from build123d import *

# Parameters (mm, degrees)
F0_W     = 5.7972974144
F0_H     = 5.9
F0_H_2   = 19.1
F1_DEPTH = 12.5
F3_D     = 4.4
F3_DEPTH = 14.1
F3_TIP   = 1.3218933619
F4_DEPTH = 3.625


with BuildPart() as f1:
    # F0 (on Front) → F1 (new body, symmetric)
    with BuildSketch(Plane.XZ):
        with Locations((-4.0329019539, -17.188550967)):
            Rectangle(F0_W, F0_H)
        with BuildLine():
            ThreePointArc((29.8217841377, -15.618166969), (29.3859073845, -15.4145662467), (28.9485841576, -15.214091327))
            ThreePointArc((28.9485841576, -15.214091327), (29.3823237659, -15.4223103801), (29.8217841377, -15.618166969))
        make_face()
        with Locations((-4.0329019539, 25.311449033)):
            Rectangle(F0_W, F0_H_2)
        with BuildLine():
            Line((19.5255004201, 0), (-1.1342532467, 0))
            Line((-1.1342532467, 0), (-1.1342532467, -9.2409374192))
            ThreePointArc((-1.1342532467, -9.2409374192), (14.2525091884, -10.4882457176), (28.9485841576, -15.214091327))
            ThreePointArc((28.9485841576, -15.214091327), (22.072081358, -8.9479478378), (19.5255004201, 0))
        make_face()
        with BuildLine():
            Line((23.5255004201, 0), (19.5255004201, 0))
            ThreePointArc((19.5255004201, 0), (22.072081358, -8.9479478378), (28.9485841576, -15.214091327))
            ThreePointArc((28.9485841576, -15.214091327), (29.3859073845, -15.4145662467), (29.8217841377, -15.618166969))
            ThreePointArc((29.8217841377, -15.618166969), (45.8723890611, -14.1878546071), (53.5125784245, 0))
            Line((53.5125784245, 0), (49.5125784245, 0))
            ThreePointArc((49.5125784245, 0), (36.5190394223, -12.9935390022), (23.5255004201, 0))
        make_face()
        Polygon((-1.1342532467, 15.761449033), (-6.9315506611, 15.761449033), (-6.9315506611, -14.238550967), (-1.1342532467, -14.238550967), (-1.1342532467, -9.2409374192), (-1.1342532467, 0), align=None)
    extrude(amount=F1_DEPTH, both=True)

    # F3
    with Locations(Plane(origin=(-6.9315506611, 0, 0), x_dir=(0, -1, 0), z_dir=(-1, 0, 0))):
        with Locations((0, 15.79714939), (0, -14.253873378)):
            Hole(F3_D / 2, depth=F3_DEPTH)
            with Locations((0, 0, -(F3_DEPTH + F3_TIP / 2))):  # 118° drill point
                Cone(0, F3_D / 2, F3_TIP, mode=Mode.SUBTRACT)

    # F0 (on Front) → F4 (join, symmetric)
    with BuildSketch(Plane.XZ):
        Polygon((-10.9315506611, 34.861449033), (-6.9315506611, 34.861449033), (-1.1342532467, 34.861449033), (-6.9315506611, 60.7583903916), (-14.991494827, 60.7583903916), (-14.991494827, 56.861449033), (-10.9315506611, 56.861449033), align=None)
    extrude(amount=F4_DEPTH, both=True)


solid = f1.part
Here's how the part is built. I have some questions about the finished solid (model axes, mm). A direction names the side the tool comes from. Coordinates: 2 decimals unless noted, no trailing zeros. Loops run counter-clockwise (first coordinate to the right, second up) from the corner with the lowest first, then second, coordinate; pieces in that order, holes last.
1. Imagine slicing it at C-C, the plane x = -3. Please give me the cut outline in (y, z) (3 decimals), and give its area (3 significant figures).
2. For faces 4 (the flat face through (-1.134, -3, 17)), 5 (the flat face through (-6.932, 0, 8)), 6 (the flat face through (-8, -3.625, 48)), which set-ups out of +Z, -Z, +X, -X, +Y, -Y let a thin tool reach every point of the face, with its end or its side?
3. If we mould it in two halves opening along Z, with no side actions, what happens to faces 1 (the flat face through (-4, 0, -20.139)), 2 (the flat face through (-1.134, 0, -17)), 3 (the cylindrical face through (-3.992, -0.286, 17.978))? For each: pulls with the +Z half, pulls with the -Z half, needs draft (parallel to the pull), parting line crosses it, or undercut.
4. Imagine slicing it at A-A, the plane y = 0. Please give me the cut outline in (x, z).
5. For P1, Ø1, axis at x = 42.5, y = 3.5, coming from the -Z side; P2, Ø1.7, axis at x = -4.5, y = 6, coming from the +Z side; P3, Ø3, axis at x = 51, y = 3, coming from the +Z side, each with a flat end and sliding along its axis, tell me the tip position at first contact or that it passes through.
6. I need wall thicknesses on L1, parallel to X at y = 5, z = 12; L2, parallel to Y at x = -4.5, z = 49.5 (3 decimals); L3, parallel to X at y = -5.75, z = -7. Which ranges of each line are inside material? Lowest first, please.
7. Imagine slicing it at D-D, the plane z = 36. Please give me the cut outline in (x, y) (3 decimals), and give its area (3 significant figures).
8. Imagine slicing it at B-B, the plane y = 7.5. Please give me the cut outline in (x, z), and give its area (3 significant figures).
Taken from the geometry:
1. outline: (-12.5, -20.139) - (12.5, -20.139) - (12.5, 34.861) - (3.625, 34.861) - (3.625, 43.196) - (-3.625, 43.196) - (-3.625, 34.861) - (-12.5, 34.861) - close; hole circle Ø4.4 at (0, -14.254); hole circle Ø4.4 at (0, 15.797)
1. area: 1,410 mm2
2. face 4: +Z, +X, +Y, -Y
2. face 5: -Z, -X, +Y, -Y
2. face 6: +Z, +X, -X, -Y
3. face 1: pulls with the -Z half
3. face 2: needs draft
3. face 3: undercut
4. outline: (-14.99, 56.86) - (-10.93, 56.86) - (-10.93, 34.86) - (-6.93, 34.86) - (-6.93, 18) - (-1.13, 18) - (-1.13, 34.86) - (-6.93, 60.76) - (-14.99, 60.76) - close; (-6.93, -20.14) - (-1.13, -20.14) - (-1.13, -16.45) - (-6.93, -16.45) - close; (-6.93, -12.05) - (-1.13, -12.05) - (-1.13, -9.24) arc R67.2 cw to (28.95, -15.21) arc R16.99 ccw to (53.51, 0) - (49.51, 0) arc R12.99 cw to (23.53, 0) - (-1.13, 0) - (-1.13, 13.6) - (-6.93, 13.6) - close
5. P1: stops at z = -16.09
5. P2: stops at z = 34.86
5. P3: stops at z = 0
6. L1: x = -6.93 to -1.13
6. L2: y = -3.625 to 3.625
6. L3: x = -6.93 to 25.57, 47.47 to 52
7. outline: (-10.932, -3.625) - (-1.389, -3.625) - (-1.389, 3.625) - (-10.932, 3.625) - close
7. area: 69.2 mm2
8. outline: (-6.93, -20.14) - (-1.13, -20.14) - (-1.13, -9.24) arc R67.2 cw to (28.95, -15.21) arc R16.99 ccw to (53.51, 0) - (49.51, 0) arc R12.99 cw to (23.53, 0) - (-1.13, 0) - (-1.13, 34.86) - (-6.93, 34.86) - close
8. area: 736 mm2
